Here's how the part is built. I have some questions about the finished solid (model axes, mm). A direction names the side the tool comes from. Round coordinates to 2 decimals unless told otherwise and drop trailing zeros. Write each loop counter-clockwise with the first axis right and the second up, starting at its lowest first coordinate (ties: lowest second). Pieces come first, ordered by that corner, then holes. Notation, with made-up numbers: (70.5, -29) -> (96.5, -29) arc R27 cw to (96.5, -3) -> close; hole circle Ø9 at (72, 66). An arc over 180 degrees is marked (long way). Answer in a Markdown table with one row per item. Add a question column.
from build123d import *

# Parameters (mm, degrees)
PAD_DEPTH = 20


with BuildPart() as part:
    # Sketch → Pad (new body)
    with BuildSketch(Plane.XY):
        Polygon((3.421999, 11), (3.421999, 9.5), (6.421999, 11), (6.421999, 13), (-7.578001, 13), (-7.578001, 0), (-4.578001, 0), (-4.578001, 11), align=None)
    pad = extrude(amount=PAD_DEPTH)

    # Mirrored: Pad across Sketch H_Axis
    add(pad.mirror(Plane.ZX))


solid = part.part
Item 1: If we section it at C-C on x = 4.5: Please give me the cut outline in (y, z), then the cut area to 3 significant figures.
Item 2: If we section it at A-A on x = 1: Please give me the cut outline in (y, z).
Item 3: If we section it at B-B on z = 14: Please give me the cut outline in (x, y).
Item 4: I need wall thicknesses on line 1 along Y through (x, z) = (-1.5, 10.5); line 2 along X through (y, z) = (-6.5, 12); line 3 along Y through (x, z) = (4.5, 7.5). Which ranges of each line are inside material? Lowest first, please. Write a range as from..to.
Item 5: If we mould it in two halves opening along Y, with no side actions, what happens to faces 4 (the flat face through (4.9, 10.24, 9.86)), 5 (the flat face through (-1, 11, 10)), 6 (the flat face through (6.422, 12, 10)), 7 (the flat face through (0, 13, 10))? For each: pulls with the +Y half, pulls with the -Y half, needs draft (parallel to the pull), parting line crosses it, or undercut.
Item 6: On a 3-axis mill with a long thin cutter (end or side, diameter ignored), from which of +Z, -Z, +X, -X, +Y, -Y can I reach the whole of each face in a straight line? I mean faces 1 (the flat face through (3.422, -10, 10)), 2 (the flat face through (4.9, -10.24, 9.86)), 3 (the flat face through (-7.578, 0, 10)). Say none if no direction works.
Item 7: If we section it at D-D on y = 3.25: Please give me the cut outline in (x, z).
Item 8: For P1, Ø4, axis at x = 0, y = 8.5, coming from the +Z side; P2, Ø10, axis at y = -3.5, z = 14, coming from the +X side, each with a flat end and sliding along its axis, tell me the tip position at first contact or that it passes through.
Results list:
| question | item | result |
|---|---|---|
| 1 | outline | (-13, 0) -> (-10.04, 0) -> (-10.04, 20) -> (-13, 20) -> close; (10.04, 0) -> (13, 0) -> (13, 20) -> (10.04, 20) -> close |
| 1 | area | 118 mm² |
| 2 | outline | (-13, 0) -> (-11, 0) -> (-11, 20) -> (-13, 20) -> close; (11, 0) -> (13, 0) -> (13, 20) -> (11, 20) -> close |
| 3 | outline | (-7.58, -13) -> (6.42, -13) -> (6.42, -11) -> (3.42, -9.5) -> (3.42, -11) -> (-4.58, -11) -> (-4.58, 11) -> (3.42, 11) -> (3.42, 9.5) -> (6.42, 11) -> (6.42, 13) -> (-7.58, 13) -> close |
| 4 | line 1 | -13..-11, 11..13 |
| 4 | line 2 | -7.58..-4.58 |
| 4 | line 3 | -13..-10.04, 10.04..13 |
| 5 | face 4 | undercut |
| 5 | face 5 | undercut |
| 5 | face 6 | needs draft |
| 5 | face 7 | pulls with the +Y half |
| 6 | face 1 | +Z, -Z |
| 6 | face 2 | +Z, -Z, +X |
| 6 | face 3 | +Z, -Z, -X, +Y, -Y |
| 7 | outline | (-7.58, 0) -> (-4.58, 0) -> (-4.58, 20) -> (-7.58, 20) -> close |
| 8 | P1 | through |
| 8 | P2 | x = -4.58 |
